```python
from build123d import *

# Parameters (mm, degrees)
SKETCH1_W            = 123
SKETCH1_H            = 72
BOSS_EXTRUDE1_DEPTH  = 2
SKETCH2_W            = 6
SKETCH2_H            = 9
BOSS_EXTRUDE2_DEPTH  = 3
SKETCH3_W            = 15
SKETCH3_H            = 9
BOSS_EXTRUDE3_DEPTH  = 5
SKETCH4_W            = 3.5
SKETCH4_H            = 9
BOSS_EXTRUDE4_DEPTH  = 6
SKETCH5_R            = 4.5
BOSS_EXTRUDE5_DEPTH  = 11.5
SKETCH6_W            = 15
SKETCH6_H            = 13
BOSS_EXTRUDE6_DEPTH  = 8
SKETCH7_W            = 26
SKETCH7_H            = 3
SKETCH7_W_2          = 21
SKETCH7_W_3          = 3
SKETCH7_H_2          = 8
SKETCH7_W_4          = 16
SKETCH7_W_5          = 5
SKETCH7_H_3          = 13
BOSS_EXTRUDE7_DEPTH  = 9
SKETCH8_W            = 12
SKETCH8_H            = 12
BOSS_EXTRUDE8_DEPTH  = 2
SKETCH9_W            = 4
SKETCH9_H            = 5
BOSS_EXTRUDE9_DEPTH  = 2
SKETCH11_W           = 7
SKETCH11_H           = 3
BOSS_EXTRUDE11_DEPTH = 8
SKETCH12_W           = 15.5
SKETCH12_H           = 1.85
BOSS_EXTRUDE12_DEPTH = 1
SKETCH13_R           = 2.54
CUT_EXTRUDE1_DEPTH   = 10


with BuildPart() as part:
    # Sketch1 → Boss-Extrude1 (new body)
    with BuildSketch(Plane(origin=(0, 0, 0), x_dir=(1, 0, 0), z_dir=(0, 1, 0))):
        Rectangle(SKETCH1_W, SKETCH1_H)
    extrude(amount=BOSS_EXTRUDE1_DEPTH)

    # Sketch2 → Boss-Extrude2 (add)
    with BuildSketch(Plane(origin=(0, 2, 0), x_dir=(1, 0, 0), z_dir=(0, 1, 0))):
        with Locations((59.5, -28.5)):
            Rectangle(SKETCH2_W, SKETCH2_H)
        with Locations((59.5, -13)):
            Rectangle(SKETCH2_W, SKETCH2_H)
    extrude(amount=BOSS_EXTRUDE2_DEPTH)

    # Sketch3 → Boss-Extrude3 (add)
    with BuildSketch(Plane(origin=(0, 2, 0), x_dir=(1, 0, 0), z_dir=(0, 1, 0))):
        with Locations((58, 28)):
            Rectangle(SKETCH3_W, SKETCH3_H)
    extrude(amount=BOSS_EXTRUDE3_DEPTH)

    # Sketch4 → Boss-Extrude4 (add)
    with BuildSketch(Plane(origin=(0, 7, 0), x_dir=(1, 0, 0), z_dir=(0, 1, 0))):
        with Locations((63.75, 28)):
            Rectangle(SKETCH4_W, SKETCH4_H)
    extrude(amount=BOSS_EXTRUDE4_DEPTH)

    # Sketch5 → Boss-Extrude5 (add)
    with BuildSketch(Plane.ZY.offset(-62)):
        with Locations((-28, 8)):
            Circle(SKETCH5_R)
    extrude(amount=BOSS_EXTRUDE5_DEPTH)

    # Sketch6 → Boss-Extrude6 (add)
    with BuildSketch(Plane(origin=(0, 2, 0), x_dir=(1, 0, 0), z_dir=(0, 1, 0))):
        with Locations((59, 12.5)):
            Rectangle(SKETCH6_W, SKETCH6_H)
    extrude(amount=BOSS_EXTRUDE6_DEPTH)

    # Sketch7 → Boss-Extrude7 (add)
    with BuildSketch(Plane(origin=(0, 2, 0), x_dir=(1, 0, 0), z_dir=(0, 1, 0))):
        with Locations((29.5, -24)):
            Rectangle(SKETCH7_W, SKETCH7_H)
        with Locations((5, -24)):
            Rectangle(SKETCH7_W_2, SKETCH7_H)
        with Locations((27, 24)):
            Rectangle(SKETCH7_W_2, SKETCH7_H)
        with Locations((36, 13)):
            Rectangle(SKETCH7_W_3, SKETCH7_H_2)
        with Locations((6, 24)):
            Rectangle(SKETCH7_W_4, SKETCH7_H)
        with Locations((27, 13)):
            Rectangle(SKETCH7_W_3, SKETCH7_H_2)
        with Locations((-6, -1)):
            Rectangle(SKETCH7_W_5, SKETCH7_H_2)
        with Locations((-19, -18.5)):
            Rectangle(SKETCH7_W_3, SKETCH7_H_3)
        with Locations((-22.1, -22.5)):
            Rectangle(SKETCH7_W_3, SKETCH7_H_3)
    extrude(amount=BOSS_EXTRUDE7_DEPTH)

    # Sketch8 → Boss-Extrude8 (add)
    with BuildSketch(Plane(origin=(0, 2, 0), x_dir=(1, 0, 0), z_dir=(0, 1, 0))):
        with Locations((-24.5, 29)):
            Rectangle(SKETCH8_W, SKETCH8_H)
    extrude(amount=BOSS_EXTRUDE8_DEPTH)

    # Sketch9 → Boss-Extrude9 (add)
    with BuildSketch(Plane(origin=(0, 2, 0), x_dir=(1, 0, 0), z_dir=(0, 1, 0))):
        with Locations((-42, 30)):
            Rectangle(SKETCH9_W, SKETCH9_H)
        with Locations((-49.5, 30)):
            Rectangle(SKETCH9_W, SKETCH9_H)
        with Locations((-57, 30)):
            Rectangle(SKETCH9_W, SKETCH9_H)
        with Locations((-34.5, 30)):
            Rectangle(SKETCH9_W, SKETCH9_H)
    extrude(amount=BOSS_EXTRUDE9_DEPTH)

    # Sketch11 → Boss-Extrude11 (add)
    with BuildSketch(Plane(origin=(0, 2, 0), x_dir=(1, 0, 0), z_dir=(0, 1, 0))):
        with Locations((-25, 6.5)):
            Rectangle(SKETCH11_W, SKETCH11_H)
    extrude(amount=BOSS_EXTRUDE11_DEPTH)

    # Sketch12 → Boss-Extrude12 (add)
    with BuildSketch(Plane(origin=(0, 2, 0), x_dir=(1, 0, 0), z_dir=(0, 1, 0))):
        with Locations((-37.75, -26.075)):
            Rectangle(SKETCH12_W, SKETCH12_H)
    extrude(amount=BOSS_EXTRUDE12_DEPTH)

    # Sketch13 → Cut-Extrude1 (cut)
    with BuildSketch(Plane(origin=(0, 2, 0), x_dir=(1, 0, 0), z_dir=(0, 1, 0))):
        with Locations((-54, -28.5)):
            Circle(SKETCH13_R)
        with Locations((-54, 22.5)):
            Circle(SKETCH13_R)
        with Locations((44.5, 23.5)):
            Circle(SKETCH13_R)
        with Locations((50, -23.5)):
            Circle(SKETCH13_R)
    extrude(amount=-CUT_EXTRUDE1_DEPTH, mode=Mode.SUBTRACT)


solid = part.part
```
Geometry: final body of the model. Coordinates: model frame, mm. A direction names the side the tool comes from. Give positions to 0.01 mm unless a question says otherwise; leave off trailing zeros. Loops run counter-clockwise (first coordinate to the right, second up) from the corner with the lowest first, then second, coordinate; pieces in that order, holes last. Notation, with made-up numbers: (40.25, -24.5) -> (62.25, -24.5) arc R6 cw to (62.25, -14.5) -> close; hole circle Ø11 at (12.5, -7.75). An arc over 180 degrees is marked (long way). Use one line per item in the form item = value.
Item 1: Line query: probe 1 along X at (y, z) = (4, -13); probe 2 along Z at (x, y) = (-54, 0.5); probe 3 along Z at (x, y) = (32, 3). Output: solid intervals per line, ascending.
A:
probe_1 = 25.5 to 28.5, 34.5 to 37.5, 51.5 to 66.5
probe_2 = -36 to -25.04, -19.96 to 25.96, 31.04 to 36
probe_3 = -25.5 to -22.5, 22.5 to 25.5
Item 2: Draft query along X for faces 1 (the face through (66.5, 6, -12)), 2 (the face through (59, 3, 24)), 3 (the face through (14, 6, -24)). Return one class per face: pulls with the +X half, pulls with the -X half, needs draft (parallel to the pull), parting line crosses it, or undercut.
A:
face_1 = pulls with the +X half
face_2 = needs draft
face_3 = undercut
Item 3: Pin query (flat end, axial travel): P1, Ø1.6, axis at y = 3, z = -29.5, coming from the +X side; P2, Ø3.5, axis at x = 59, y = 4, coming from the +Z side; P3, Ø2.5, axis at y = 8.5, z = 24, coming from the +X side. Return the tip coordinate at first contact, or that it passes through.
A:
P1 = 65.5
P2 = 33
P3 = 42.5
Item 4: Section query A-A on x = 44.5. Output: boundary loops of the cut face in (y, z).
A:
outline = (0, -36) -> (2, -36) -> (2, -26.04) -> (0, -26.04) -> close; (0, -20.96) -> (2, -20.96) -> (2, 36) -> (0, 36) -> close
Item 5: Section query B-B on x = -7. Output: boundary loops of the cut face in (y, z), and give its area (3 significant figures).
A:
outline = (0, -36) -> (2, -36) -> (2, -3) -> (11, -3) -> (11, 5) -> (2, 5) -> (2, 36) -> (0, 36) -> close
area = 216 mm^2
Item 6: Access query for faces 4 (the face through (27, 11, -24)), 5 (the face through (-19, 6, 12)), 6 (the face through (34.5, 6, -13)), 7 (the face through (59, 3, 33)). Directions: +Z, -Z, +X, -X, +Y, -Y. A direction counts if a zero-diameter tool reaches every point of the face in a straight line with its end or side. Return the directions, or none.
A:
face_4 = +Z, -Z, -X, +Y
face_5 = -X, +Y
face_6 = +Y
face_7 = +Z, +X, -X, +Y
